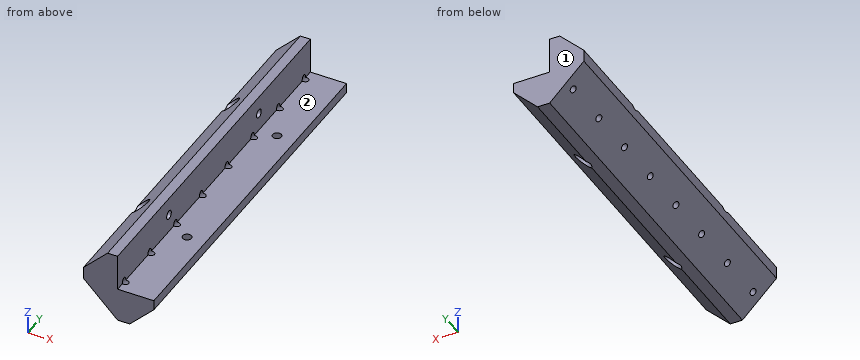
Autodesk Inventor part; units mm, degrees
ref_plane "YZ Plane" through (0, 0, 0) normal (1, 0, 0) x (0, 1, 0)
ref_plane "XZ Plane" through (0, 0, 0) normal (0, 1, 0) x (-1, 0, 0)
ref_plane "XY Plane" through (0, 0, 0) normal (0, 0, 1) x (1, 0, 0)
sketch "Sketch1" plane through (0, 0, 0) normal (0, 1, 0) x (-1, 0, 0)
  line L0 (0, 0) -> (0, 15)
  line L1 (0, 15) -> (14.1421, 15)
  line L2 (14.1421, 15) -> (14.1421, 0)
  line L3 (14.1421, 0) -> (0, -14.1421)
  line L4 (0, -14.1421) -> (-15, -14.1421)
  line L5 (-15, -14.1421) -> (-15, 0)
  line L6 (-15, 0) -> (0, 0)
  dimension "d0" = 15
  dimension "d1" = 10
extrude "Extrusion1" add sketch "Sketch1" along normal blind 150
chamfer "Chamfer1" distance 10 angle 45 2 edges at (-14.1421, 75, 15) (15, 75, -14.1421)
sketch "Sketch2" plane through (-14.1421, 0, 0) normal (-1, 0, 0) x (0, 0, 1)
  line L0 (15, 150) -> (5, 150)
  line L1 (5, 150) -> (5, 0)
  line L2 (5, 0) -> (15, 0)
  line L3 (15, 0) -> (15, 150)
  line L4 (5, 150) -> (5, 0)
  line L5 (0, 150) -> (5, 150)
  line L6 (0, 0) -> (0, 150)
  line L7 (0, 0) -> (5, 0)
  point P0 (0, 0)
  point P1 (7.5, 40)
  point P2 (7.5, 110)
  dimension "d7" = 7.5
  dimension "d8" = 40
  dimension "d9" = 40
hole "Hole1" at (-14.1421, 40, 7.5) at (-14.1421, 110, 7.5) direction (1, 0, 0) diameter 3.6 end through all counterbore diameter 6.5 counterbore depth 10
sketch "Sketch3" plane through (0, 0, -14.1421) normal (0, 0, -1) x (-1, 0, 0)
  line L0 (-5, 150) -> (-15, 150)
  line L1 (-15, 150) -> (-15, 0)
  line L2 (-15, 0) -> (-5, 0)
  line L3 (-5, 0) -> (-5, 150)
  line L4 (-5, 0) -> (-5, 150)
  line L5 (-5, 0) -> (0, 0)
  line L6 (0, 0) -> (0, 150)
  line L7 (-5, 150) -> (0, 150)
  point P0 (-7.5, 40)
  point P1 (-7.5, 110)
  dimension "d17" = 40
  dimension "d18" = 40
  dimension "d26" = 7.5
hole "Hole2" at (7.5, 40, -14.1421) at (7.5, 110, -14.1421) direction (0, 0, 1) diameter 3.6 end through all counterbore diameter 6.5 counterbore depth 10
sketch "Sketch4" plane through (-14.1421, 0, 0) normal (-0.7071, 0, -0.7071) x (-0.7071, 0, 0.7071)
  circle A0 centre (-10, 25) radius 3
  circle A1 centre (-10, 65) radius 3
  circle A2 centre (-10, 105) radius 3
  circle A3 centre (-10, 145) radius 3
  circle A4 centre (-10, 185) radius 3
  circle A5 centre (-10, 225) radius 3
  circle A6 centre (-10, 265) radius 3
  circle A7 centre (-10, 285) radius 3
  circle A8 centre (-10, 245) radius 3
  circle A9 centre (-10, 205) radius 3
  circle A10 centre (-10, 165) radius 3
  circle A11 centre (-10, 125) radius 3
  circle A12 centre (-10, 85) radius 3
  circle A13 centre (-10, 45) radius 3
  circle A14 centre (-10, 5) radius 3
  line L0 (-5.5, 290) -> (-14.5, 290)
  line L1 (-14.5, 290) -> (-14.5, -60)
  line L2 (-5.5, -60) -> (-14.5, -60)
  line L3 (-5.5, 290) -> (-5.5, -60)
  circle A15 centre (-10, -55) radius 3
  circle A16 centre (-10, -15) radius 3
  circle A17 centre (-10, -35) radius 3
  point P0 (-10, 0)
hole "Hole3" at (-7.0711, 165, -7.0711) at (-7.0711, 145, -7.0711) at (-7.0711, 125, -7.0711) at (-7.0711, 105, -7.0711) at (-7.0711, 85, -7.0711) at (-7.0711, 65, -7.0711) at (-7.0711, 45, -7.0711) at (-7.0711, 25, -7.0711) at (-7.0711, 5, -7.0711) direction (0.7071, 0, 0.7071) diameter 2.8 end through all
properties part number "Corner Z Brace" material "ABS Plastic"
Verification items for the finished model (mm, model axes). Face numbers are marked on the shaded views. A direction names the side the tool comes from. Coordinates: 2 decimals unless noted, no trailing zeros. Write each loop counter-clockwise with the first axis right and the second up, starting at its lowest first coordinate (ties: lowest second). Pieces come first, ordered by that corner, then holes. Notation, with made-up numbers: (59, 54.5) -> (118, 54.5) arc R7 cw to (118, 59.5) -> close; hole circle Ø1 at (-5.75, 68.5). An arc over 180 degrees is marked (long way). One line per item, written item: value. Start each with the question number.
Q1. Cross-section at A-A on z = 7.5. Enter the section's corners in (x, y), and give its area (3 significant figures).
Q2. Cross-section at B-B on y = 110. Enter the section's corners in (x, z).
Q3. Thickness scan on L1, parallel to Y at x = -1.95, z = 7.5; L2, parallel to Y at x = -8.25, z = 7.5; L3, parallel to X at y = 106, z = 5. Record the ranges inside material, lowest first. Write a range as from..to.
Q4. Access from +Z, -Z, +X, -X, +Y, -Y to the whole of each face (thin tool, end or side, straight path). Record for the marked faces 1 and 2.
Q5. Cross-section at D-D on y = 81.5. Enter the section's corners in (x, z), and give its area (3 significant figures).
Q6. Go/stop test with flat-tipped pins: P1, Ø2, axis at y = 46.5, z = 4.5, coming from the +X side; P2, Ø7.5, axis at x = 6, y = 48, coming from the +Z side; P3, Ø3, axis at x = 7.5, y = 110, coming from the +Z side; P4, Ø3, axis at x = 8, y = 39.5, coming from the -Z side. Record where each tip stops, or that it passes through.
Q7. Cross-section at C-C on x = 7.5. Enter the section's corners in (y, z).
Checked values:
1. outline: (-11.64, 0) -> (0, 0) -> (0, 38.2) -> (-4.14, 38.2) -> (-4.14, 36.75) -> (-11.64, 36.75) -> close; (-11.64, 43.25) -> (-4.14, 43.25) -> (-4.14, 41.8) -> (0, 41.8) -> (0, 108.2) -> (-4.14, 108.2) -> (-4.14, 106.75) -> (-11.64, 106.75) -> close; (-11.64, 113.25) -> (-4.14, 113.25) -> (-4.14, 111.8) -> (0, 111.8) -> (0, 150) -> (-11.64, 150) -> close
1. area: 1,620 mm²
2. outline: (-14.14, 0) -> (0, -14.14) -> (4.25, -14.14) -> (4.25, -4.14) -> (5.7, -4.14) -> (5.7, 0) -> (0, 0) -> (0, 5.7) -> (-4.14, 5.7) -> (-4.14, 4.25) -> (-14.14, 4.25) -> close; (-8.39, 10.75) -> (-4.14, 10.75) -> (-4.14, 9.3) -> (0, 9.3) -> (0, 15) -> (-4.14, 15) -> close; (9.3, -4.14) -> (10.75, -4.14) -> (10.75, -8.39) -> (15, -4.14) -> (15, 0) -> (9.3, 0) -> close
3. L1: y = 0..38.2, 41.8..108.2, 111.8..150
3. L2: y = 0..36.75, 43.25..106.75, 113.25..150
3. L3: x = -14.14..0
4. face 1: +Z, -Z, +X, -X, +Y
4. face 2: +Z, +X, +Y, -Y
5. outline: (-14.14, 0) -> (0, -14.14) -> (5, -14.14) -> (15, -4.14) -> (15, 0) -> (0, 0) -> (0, 15) -> (-4.14, 15) -> (-14.14, 5) -> close
5. area: 424 mm²
6. P1: stops at x = 0
6. P2: stops at z = 0
6. P3: passes through
6. P4: stops at z = -4.14
7. outline: (0, -11.64) -> (36.75, -11.64) -> (36.75, -4.14) -> (38.2, -4.14) -> (38.2, 0) -> (0, 0) -> close; (41.8, -4.14) -> (43.25, -4.14) -> (43.25, -11.64) -> (106.75, -11.64) -> (106.75, -4.14) -> (108.2, -4.14) -> (108.2, 0) -> (41.8, 0) -> close; (111.8, -4.14) -> (113.25, -4.14) -> (113.25, -11.64) -> (150, -11.64) -> (150, 0) -> (111.8, 0) -> close
